Autodesk Inventor part; units mm, degrees
ref_plane "1_XY" through (7.0739, 0, 0) normal (1, 0, 0) x (0, 0, -1)
ref_plane "1_YZ" through (7.0739, 0, 0) normal (0, 0, -1) x (0, 1, 0)
ref_plane "1_ZX" through (7.0739, 0, 0) normal (0, 1, 0) x (1, 0, 0)
sketch "Sketch_1" plane through (0, 0, 0) normal (0, 0, 1) x (1, 0, 0)
  line L0 (7.0739, 0) -> (0, 0)
  line L1 (0, 0) -> (0, 8.9091)
  line L2 (0, 8.9091) -> (0.762, 9.671)
  line L3 (0.762, 9.671) -> (2.4384, 9.671)
  line L4 (2.4384, 9.671) -> (3.2004, 8.9091)
  line L5 (3.2004, 8.9091) -> (3.9624, 8.9091)
  line L6 (3.9624, 8.9091) -> (3.9624, 10.2235)
  line L7 (3.9624, 10.2235) -> (7.0739, 10.2235)
  line L8 (7.0739, 10.2235) -> (7.0739, 0)
  line L9 (7.0739, 0) -> (0, 0)
revolve "Revolution1" add sketch "Sketch_1" angle 360 about axis through (7.0739, 0, 0) along (1, 0, 0)
sketch "Sketch_24" plane through (0, 0, 0) normal (0, 0, 1) x (1, 0, 0)
  line L0 (3.9624, 0) -> (3.2004, 0)
  line L1 (3.0477, 10.2235) -> (3.0477, 10.1393)
  line L2 (3.0477, 10.1393) -> (3.8399, 9.3472)
  arc A0 (3.8399, 9.1676) -> (3.8399, 9.3472) centre (3.7501, 9.2574) ccw
  line L3 (3.8399, 9.1676) -> (3.5814, 8.9091)
  line L4 (3.5814, 8.9091) -> (3.2004, 8.9091)
  line L5 (3.2004, 8.9091) -> (3.2004, 8.655)
  line L6 (3.2004, 8.655) -> (3.9624, 8.655)
  line L7 (3.9624, 8.655) -> (3.9624, 9.512)
  line L8 (3.9624, 9.512) -> (3.2509, 10.2235)
  line L9 (3.2509, 10.2235) -> (3.0477, 10.2235)
revolve "Revolution2" add sketch "Sketch_24" angle 360 about axis through (3.9624, 0, 0) along (1, 0, 0)
sketch "Sketch_26" plane through (0, 0, 0) normal (0, 0, 1) x (1, 0, 0)
  line L0 (0, 0) -> (-3.175, 0)
  line L1 (-3.175, 0) -> (-3.175, 6.3754)
  line L2 (-3.175, 6.3754) -> (-2.413, 7.1374)
  line L3 (-2.413, 7.1374) -> (0, 7.1374)
  line L4 (0, 7.1374) -> (0, 0)
  line L5 (0, 0) -> (-3.175, 0)
revolve "Revolution3" add sketch "Sketch_26" angle 360 about axis through (0, 0, 0) along (1, 0, 0)
sketch "Sketch_27" plane through (0, 0, 0) normal (0, 0, 1) x (1, 0, 0)
  line L0 (22.9489, 0) -> (7.0739, 0)
  line L1 (7.0739, 0) -> (7.0739, 7.9375)
  line L2 (7.0739, 7.9375) -> (22.1869, 7.9375)
  line L3 (22.1869, 7.9375) -> (22.9489, 7.1755)
  line L4 (22.9489, 7.1755) -> (22.9489, 0)
  line L5 (22.9489, 0) -> (7.0739, 0)
revolve "Revolution4" add sketch "Sketch_27" angle 360 about axis through (22.9489, 0, 0) along (1, 0, 0)
sketch "Sketch_28" plane through (7.2009, 0, 0) normal (1, 0, 0) x (0, 0, -1)
  line L0 (-15.875, 15.875) -> (-15.875, -15.875)
  line L1 (-15.875, -15.875) -> (15.875, -15.875)
  line L2 (15.875, -15.875) -> (15.875, 15.875)
  line L3 (15.875, 15.875) -> (-15.875, 15.875)
  line L4 (-12.7, 4.7308) -> (-12.7, -4.7308)
  line L5 (-12.7, -4.7308) -> (12.7, -4.7308)
  line L6 (12.7, -4.7308) -> (12.7, 4.7308)
  line L7 (12.7, 4.7308) -> (-12.7, 4.7308)
extrude "Extrusion1" cut sketch "Sketch_28" along normal blind 15.875
sketch "Sketch_29" plane through (0, 0, 0) normal (0, 1, 0) x (-1, 0, 0)
  circle A0 centre (-15.875, 0) radius 3.2004
extrude "Extrusion2" cut sketch "Sketch_29" along normal mid plane 18.923
ref_plane "1_XY" through (7.0739, 0, 0) normal (1, 0, 0) x (0, 0, -1)
ref_plane "1_YZ" through (7.0739, 0, 0) normal (0, 0, -1) x (0, 1, 0)
ref_plane "1_ZX" through (7.0739, 0, 0) normal (0, 1, 0) x (1, 0, 0)
ref_plane "lovra_XY" through (7.0739, 0, 0) normal (1, 0, 0) x (0, 1, 0)
ref_plane "lovra_YZ" through (7.0739, 0, 0) normal (0, 1, 0) x (0, 0, 1)
ref_plane "lovra_ZX" through (7.0739, 0, 0) normal (0, 0, 1) x (1, 0, 0)
ref_plane "lovra1_XY" through (2.2987, 0, 0) normal (1, 0, 0) x (0, 0, -1)
ref_plane "lovra1_YZ" through (2.2987, 0, 0) normal (0, 0, -1) x (0, 1, 0)
ref_plane "lovra1_ZX" through (2.2987, 0, 0) normal (0, 1, 0) x (1, 0, 0)
ref_plane "lovra2_XY" through (2.2987, 7.874, 0) normal (1, 0, 0) x (0, 0, -1)
ref_plane "lovra2_YZ" through (2.2987, 7.874, 0) normal (0, 0, -1) x (0, 1, 0)
ref_plane "lovra2_ZX" through (2.2987, 7.874, 0) normal (0, 1, 0) x (1, 0, 0)
ref_plane "lovra21_XY" through (0, 0, 5.2705) normal (1, 0, 0) x (0, 0, -1)
ref_plane "lovra21_YZ" through (0, 0, 5.2705) normal (0, 0, -1) x (0, 1, 0)
ref_plane "lovra21_ZX" through (0, 0, 5.2705) normal (0, 1, 0) x (1, 0, 0)
ref_plane "lovra22_XY" through (0, 0, -5.2705) normal (1, 0, 0) x (0, 0, -1)
ref_plane "lovra22_YZ" through (0, 0, -5.2705) normal (0, 0, -1) x (0, 1, 0)
ref_plane "lovra22_ZX" through (0, 0, -5.2705) normal (0, 1, 0) x (1, 0, 0)
ref_plane "lovra3_XY" through (2.2987, -7.874, 0) normal (1, 0, 0) x (0, 0, -1)
ref_plane "lovra3_YZ" through (2.2987, -7.874, 0) normal (0, 0, -1) x (0, 1, 0)
ref_plane "lovra3_ZX" through (2.2987, -7.874, 0) normal (0, 1, 0) x (1, 0, 0)
ref_plane "olen_XY" through (15.875, 0, 0) normal (1, 0, 0) x (0, 0, -1)
ref_plane "olen_YZ" through (15.875, 0, 0) normal (0, 0, -1) x (0, 1, 0)
ref_plane "olen_ZX" through (15.875, 0, 0) normal (0, 1, 0) x (1, 0, 0)
ref_plane "p1_XY" through (22.9489, 0, 4.7308) normal (1, 0, 0) x (0, 0, -1)
ref_plane "p1_YZ" through (22.9489, 0, 4.7308) normal (0, 0, -1) x (0, 1, 0)
ref_plane "p1_ZX" through (22.9489, 0, 4.7308) normal (0, 1, 0) x (1, 0, 0)
ref_plane "p2_XY" through (22.9489, 0, -4.7308) normal (1, 0, 0) x (0, 0, -1)
ref_plane "p2_YZ" through (22.9489, 0, -4.7308) normal (0, 0, -1) x (0, 1, 0)
ref_plane "p2_ZX" through (22.9489, 0, -4.7308) normal (0, 1, 0) x (1, 0, 0)
ref_plane "port2_XY" through (22.9489, 0, 0) normal (1, 0, 0) x (0, 0, -1)
ref_plane "port2_YZ" through (22.9489, 0, 0) normal (0, 0, -1) x (0, 1, 0)
ref_plane "port2_ZX" through (22.9489, 0, 0) normal (0, 1, 0) x (1, 0, 0)
ref_plane "thd1_XY" through (22.9489, 0, 7.9375) normal (1, 0, 0) x (0, 0, -1)
ref_plane "thd1_YZ" through (22.9489, 0, 7.9375) normal (0, 0, -1) x (0, 1, 0)
ref_plane "thd1_ZX" through (22.9489, 0, 7.9375) normal (0, 1, 0) x (1, 0, 0)
ref_plane "thd2_XY" through (22.9489, 0, -7.9375) normal (1, 0, 0) x (0, 0, -1)
ref_plane "thd2_YZ" through (22.9489, 0, -7.9375) normal (0, 0, -1) x (0, 1, 0)
ref_plane "thd2_ZX" through (22.9489, 0, -7.9375) normal (0, 1, 0) x (1, 0, 0)
ref_plane "to_mounting_bracket_XY" through (23.0124, 0, 0) normal (1, 0, 0) x (0, 0, -1)
ref_plane "to_mounting_bracket_YZ" through (23.0124, 0, 0) normal (0, 0, -1) x (0, 1, 0)
ref_plane "to_mounting_bracket_ZX" through (23.0124, 0, 0) normal (0, 1, 0) x (1, 0, 0)
ref_plane "to_nut_XY" through (25.4, 0, 0) normal (1, 0, 0) x (0, 0, -1)
ref_plane "to_nut_YZ" through (25.4, 0, 0) normal (0, 0, -1) x (0, 1, 0)
ref_plane "to_nut_ZX" through (25.4, 0, 0) normal (0, 1, 0) x (1, 0, 0)
ref_plane "to_pin_XY" through (15.875, 0, 0) normal (0, 1, 0) x (1, 0, 0)
ref_plane "to_pin_YZ" through (15.875, 0, 0) normal (1, 0, 0) x (0, 0, -1)
ref_plane "to_pin_ZX" through (15.875, 0, 0) normal (0, 0, -1) x (0, 1, 0)
ref_plane "to_pin_1_XY" through (15.875, 0, 0) normal (0, 0, 1) x (1, 0, 0)
ref_plane "to_pin_1_YZ" through (15.875, 0, 0) normal (1, 0, 0) x (0, 1, 0)
ref_plane "to_pin_1_ZX" through (15.875, 0, 0) normal (0, 1, 0) x (0, 0, 1)
ref_plane "to_pin_r_XY" through (15.875, 0, 0) normal (0, 0, 1) x (1, 0, 0)
ref_plane "to_pin_r_YZ" through (15.875, 0, 0) normal (1, 0, 0) x (0, 1, 0)
ref_plane "to_pin_r_ZX" through (15.875, 0, 0) normal (0, 1, 0) x (0, 0, 1)
ref_plane "to_screw_XY" through (17.4752, -6.0452, -2.032) normal (0, 0, -1) x (1, 0, 0)
ref_plane "to_screw_YZ" through (17.4752, -6.0452, -2.032) normal (1, 0, 0) x (0, -1, 0)
ref_plane "to_screw_ZX" through (17.4752, -6.0452, -2.032) normal (0, -1, 0) x (0, 0, -1)
ref_plane "to_tube_XY" through (3.2004, 0, 0) normal (1, 0, 0) x (0, 0, -1)
ref_plane "to_tube_YZ" through (3.2004, 0, 0) normal (0, 0, -1) x (0, 1, 0)
ref_plane "to_tube_ZX" through (3.2004, 0, 0) normal (0, 1, 0) x (1, 0, 0)
properties part number "04PR0K000_rear_head"
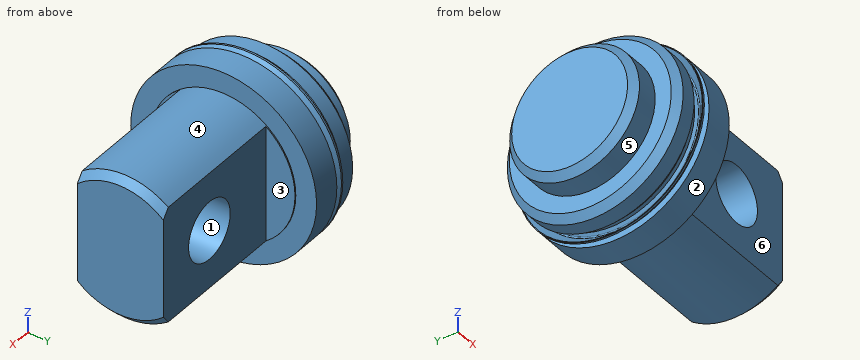
The listing builds one solid part. Answer for the finished solid, in the listing's coordinates (mm). Face numbers are marked on the shaded views. A direction names the side the tool comes from. Coordinates: 2 decimals unless noted, no trailing zeros. Order: outer loops, then holes, each group sorted by start corner. A loop starts at its lowest first (then second) coordinate and runs counter-clockwise, first axis right, second up. Notation, with made-up numbers: (50.25, -23) -> (108.25, -23) arc R9 ccw to (108.25, -17) -> close; hole circle Ø9 at (8, -39.5). An arc over 180 degrees is marked (long way). Answer in a Markdown table with one row per item. Add a question column.
Item 1: Find the intervals of material crossed by L1, parallel to X at y = 2.75, z = 0 (3 decimals); L2, parallel to Y at x = 3.75, z = 0.5; L3, parallel to X at y = -2, z = -9, in increasing order. Write a range as from..to.
Item 2: Determine the mould class of the marked faces 1, 2 and 3 for opening direction Z: +Z half, -Z half, draft (parallel to the pull), parting line (faces both ways), or undercut.
Item 3: Find section B-B (x = 2). Write down the section's boundary in (y, z).
Item 4: Which of the six approach directions +Z, -Z, +X, -X, +Y, -Y give full straight-line access (tool end or side, diameter ignored) to the marked faces 4, 5 and 6?
Item 5: Each of these flat-tipped pins is pushed along its axis until it touches: P1, Ø2, axis at x = 6, y = 3.5, coming from the -Z side; P2, Ø1, axis at y = -6, z = -3, coming from the +X side; P3, Ø10, axis at x = 16, z = -1, coming from the +Y side; P4, Ø4, axis at x = 15.875, z = 0, coming from the +Y side. Where does it stop, or does it pass through?
Item 6: Find section A-A (x = 14.5). Write down the section's boundary in (y, z) (1 decimal).
Result set:
| question | item | result |
|---|---|---|
| 1 | L1 | x = -3.175..12.675, 19.075..22.949 |
| 1 | L2 | y = -9.71..-9.42, -9.06..9.06, 9.42..9.71 |
| 1 | L3 | x = 0.31..2.89, 3.87..7.07 |
| 2 | face 1 | undercut |
| 2 | face 2 | parting line |
| 2 | face 3 | draft |
| 3 | outline | circle Ø19.34 at (0, 0) |
| 4 | face 4 | +X |
| 4 | face 5 | -X |
| 4 | face 6 | +Z, -Z, +X, -Y |
| 5 | P1 | stops at z = -9.91 |
| 5 | P2 | stops at x = 7.2 |
| 5 | P3 | stops at y = 4.73 |
| 5 | P4 | passes through |
| 6 | outline | (-4.7, -6.4) arc R7.9 ccw to (4.7, -6.4) -> (4.7, -2.9) -> (-4.7, -2.9) -> close; (-4.7, 2.9) -> (4.7, 2.9) -> (4.7, 6.4) arc R7.9 ccw to (-4.7, 6.4) -> close |
